```python
from build123d import *


with BuildPart() as part:
    # Sketch2 → Revolve4 (revolve)
    with BuildSketch(Plane(origin=(0, 0, 0), x_dir=(1, 0, 0), z_dir=(0, 1, 0))):
        Polygon((24.882765403, 17.005709542), (25.875695003, -55.987537343), (29.626041942, -55.987537343), (29.605639279, -54.487676105), (28.580544449, -54.487676105), (28.485332021, -47.488323664), (28.860366715, -47.488323664), (27.97160056, 17.8475545), (27.163610623, 17.8475545), (25.134414226, 43.778408192), (24.518575479, 43.778408192), align=None)
    revolve(axis=Axis((24.882765403, 0, -17.005709542), (0.013601775, 0, 0.999907492)))


solid = part.part
```
The model under review builds one solid part; all positions refer to its coordinate system, in mm. Round coordinates to 2 decimals unless told otherwise and drop trailing zeros. Use CSV: the item, a comma, the result in double quotes. Start each with the question number.
(1) The part is to be moulded in two halves that separate along Z. For faces 1 (the face through (22.85, -1.886, 14.439)), 2 (the face through (23.252, 0.063, -30.955)), 3 (the face through (26.092, -0.09, 55.988)), say which applies: +Z half, -Z half, draft (parallel to the pull), parting line (faces both ways), or undercut.
(2) Clearance check with flat-ended pins moving along their axes: P1, Ø3, axis at y = -2, z = -10.5, coming from the -X side; P2, Ø2, axis at x = 23.5, y = 1.5, coming from the +Z side; P3, Ø4, axis at y = 2.5, z = 35.5, coming from the -X side. State where each tip first meets the part, or that it passes through.
(3) For line 1 along Z through (x, y) = (27.75, 2.5); line 2 along Y through (x, z) = (25.5, 18); line 3 along Z through (x, y) = (24, -2.5), list the stretches that pass through material, from the lowest coordinate up.
Findings:
1,face 1,"undercut"
1,face 2,"-Z half"
1,face 3,"+Z half"
2,P1,"x = 21.91"
2,P2,"z = 56.08"
2,P3,"x = 22.54"
3,line 1,"54.5 to 56"
3,line 2,"-3.1 to 3.1"
3,line 3,"-17.8 to 47.55, 54.56 to 56.06"
